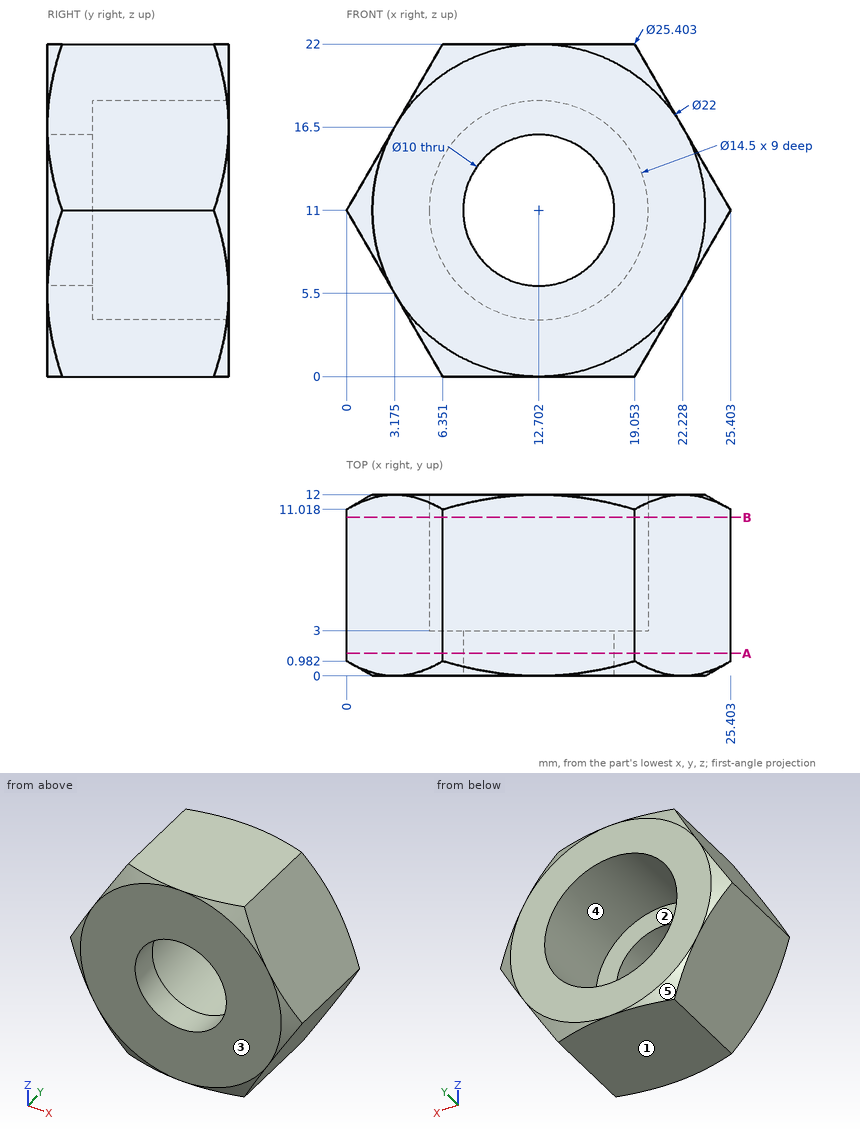
Drawing for the job (mm, zero at the part's lowest x, y, z). A direction names the side the tool comes from. Round coordinates to 2 decimals unless told otherwise and drop trailing zeros. Order: outer loops, then holes, each group sorted by start corner. A loop starts at its lowest first (then second) coordinate and runs counter-clockwise, first axis right, second up. Notation, with made-up numbers: (39, -0.75) -> (61, -0.75) arc R34 cw to (61, 32.25) -> close; hole circle Ø2 at (4.5, 4). An arc over 180 degrees is marked (long way). Put each result on its own line as item: value.
Q1. Wall check: line 1 (Z direction, x = 12.5, y = 0.5) (1 decimal); line 2 (Z direction, x = 8.5, y = 2); line 3 (Y direction, x = 17.25, z = 6.75). Give the ranges that are in metal, low to high. Write a range as [from, to].
From the geometry:
line 1: z = [0, 6], [16, 22]
line 2: z = [0, 8.29], [13.71, 22]
line 3: y = [0, 3]
Q2. Pin check, flat tip, straight feed: pin 1 Ø7 at (x, z) = (14, 12) entering from +Y. Stop position of the tip, or through.
From the geometry:
pin 1: stops at y = 3
Q3. Pull direction Z, two halves, no side cores. Call the marked faces 3, 4 and 5: pulls with the +Z half, pulls with the -Z half, needs draft (parallel to the pull), parting line crosses it, or undercut.
From the geometry:
face 3: needs draft
face 4: undercut
face 5: pulls with the -Z half
Q4. Band-saw the part on A-A (y = 1.5). Give the cut face in (x, z).
From the geometry:
outline: (0, 11) -> (6.35, 0) -> (19.05, 0) -> (25.4, 11) -> (19.05, 22) -> (6.35, 22) -> close; hole circle Ø10 at (12.7, 11)
Q5. Tool access for the marked faces 1 and 2: list every direction of +Z, -Z, +X, -X, +Y, -Y with a clear straight run to the whole face (end or side of a thin tool).
From the geometry:
face 1: -Z, +X, -X, +Y, -Y
face 2: +Y
Q6. Band-saw the part on B-B (y = 10.5). Give the cut face in (x, z), and give its area (3 significant figures).
From the geometry:
outline: (0, 11) -> (6.35, 0) -> (19.05, 0) -> (25.4, 11) -> (19.05, 22) -> (6.35, 22) -> close; hole circle Ø14.5 at (12.7, 11)
area: 254 mm2
